Design review of the part shown in the three views and the two pictorial views. Dimensions are in mm from the part's minimum x, y and z. A direction names the side the tool comes from. Coordinates: 2 decimals unless noted, no trailing zeros. Write each loop counter-clockwise with the first axis right and the second up, starting at its lowest first coordinate (ties: lowest second). Pieces come first, ordered by that corner, then holes. Notation, with made-up numbers: M 22,29.5 L 41,29.5 A23 cw 41,63.5 Z; hole C 20.25,-5 d7. An arc over 180 degrees is marked long. One line per question, with ' | ' between items.
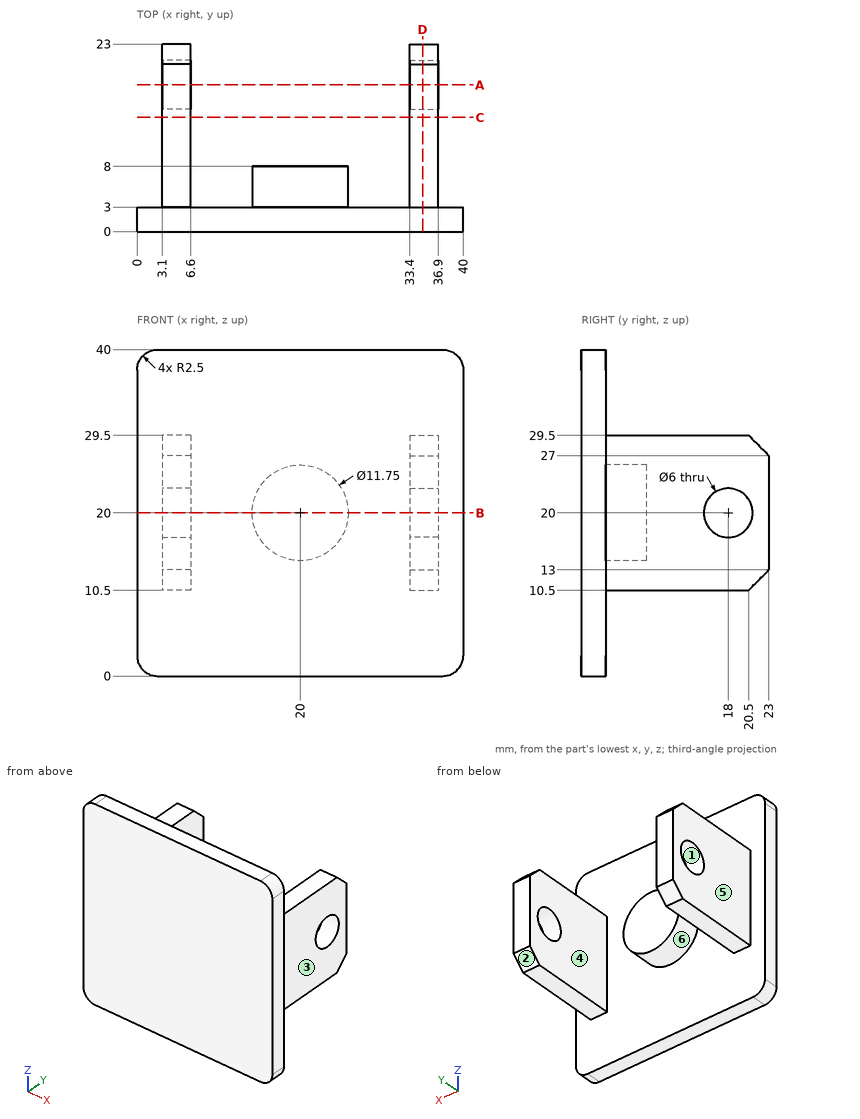
1. Take a section at C-C on y = 14. State the section outline as (x, z) points, plus the area to 3 significant figures.
Computed values:
outline: M 3.1,10.5 L 6.6,10.5 L 6.6,29.5 L 3.1,29.5 Z; M 33.4,10.5 L 36.9,10.5 L 36.9,29.5 L 33.4,29.5 Z | area: 133 mm2
2. Take a section at A-A on y = 18. State the section outline as (x, z) points.
Computed values:
outline: M 3.1,10.5 L 6.6,10.5 L 6.6,17 L 3.1,17 Z; M 3.1,23 L 6.6,23 L 6.6,29.5 L 3.1,29.5 Z; M 33.4,10.5 L 36.9,10.5 L 36.9,17 L 33.4,17 Z; M 33.4,23 L 36.9,23 L 36.9,29.5 L 33.4,29.5 Z
3. For line 1 along X through (y, z) = (13.25, 22.5); line 2 along Y through (x, z) = (34, 20); line 3 along Y through (x, z) = (35.5, 30.5), list the stretches that pass through material, from the lowest coordinate up.
Computed values:
line 1: x = 3.1 to 6.6, 33.4 to 36.9 | line 2: y = 0 to 15, 21 to 23 | line 3: y = 0 to 3
4. Take a section at D-D on x = 35. State the section outline as (y, z) points, plus the area to 3 significant figures.
Computed values:
outline: M 0,0 L 3,0 L 3,10.5 L 20.5,10.5 L 23,13 L 23,27 L 20.5,29.5 L 3,29.5 L 3,40 L 0,40 Z; hole C 18,20 d6 | area: 465 mm2
5. Machinability: for the marked faces 4, 5 and 6, which of the approach directions +Z, -Z, +X, -X, +Y, -Y give a long, thin tool a straight path to every point of the face, cutting with its end or side? Answer none if there is none.
Computed values:
face 4: +Z, -Z, +Y | face 5: +Z, -Z, -X, +Y | face 6: +Y
6. Take a section at B-B on z = 20. State the section outline as (x, y) points (3 decimals).
Computed values:
outline: M 0,0 L 40,0 L 40,3 L 36.9,3 L 36.9,15 L 33.4,15 L 33.4,3 L 25.875,3 L 25.875,8 L 14.125,8 L 14.125,3 L 6.6,3 L 6.6,15 L 3.1,15 L 3.1,3 L 0,3 Z; M 3.1,21 L 6.6,21 L 6.6,23 L 3.1,23 Z; M 33.4,21 L 36.9,21 L 36.9,23 L 33.4,23 Z
7. Clearance check with flat-ended pins moving along their axes: P1, Ø3, axis at x = 31, z = 19.5, coming from the +Y side; P2, Ø1, axis at x = 34.5, y = 13, coming from the -Z side; P3, Ø3, axis at x = 5, y = 13, coming from the +Z side. State where each tip first meets the part, or that it passes through.
Computed values:
P1: stops at y = 3 | P2: stops at z = 10.5 | P3: stops at z = 29.5
8. Draft analysis for pull direction Y (two halves, no side actions). For the marked faces 1, 2 and 3, state which applies: pulls with the +Y half, pulls with the -Y half, needs draft (parallel to the pull), parting line crosses it, or undercut.
Computed values:
face 1: undercut | face 2: pulls with the +Y half | face 3: needs draft
